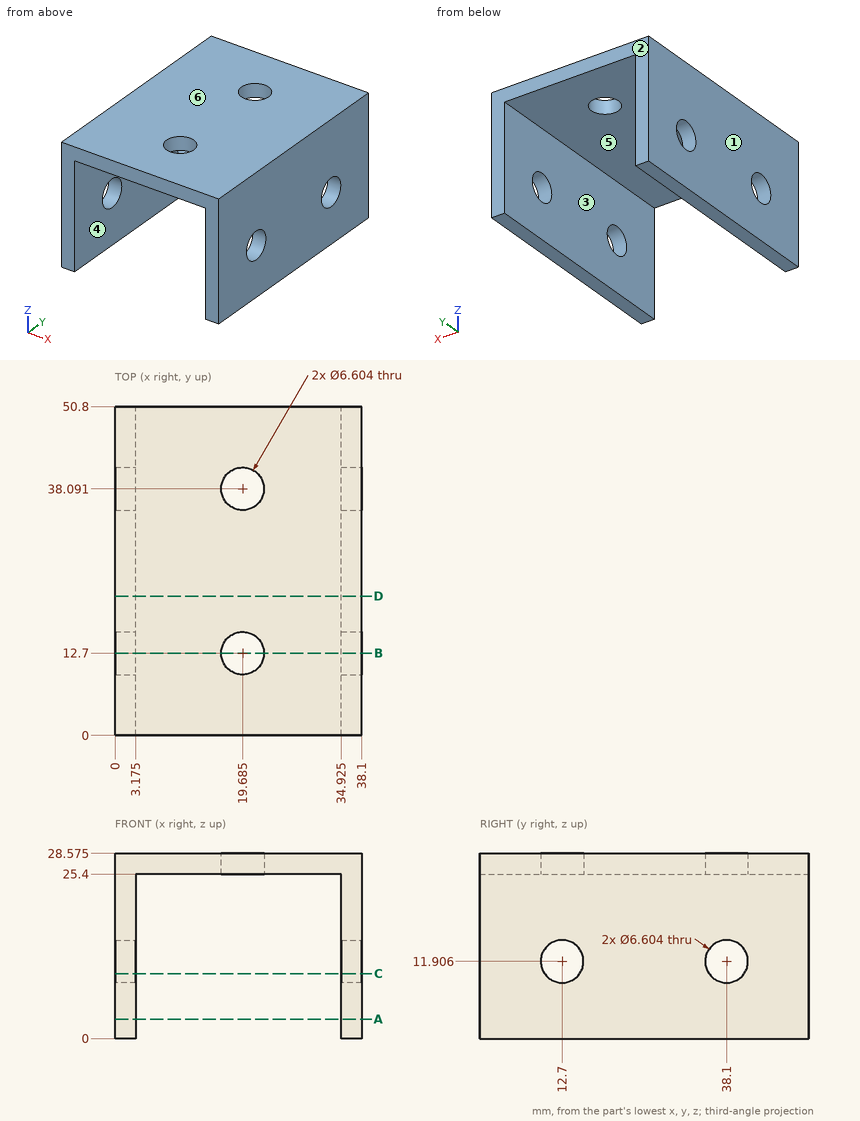
Verification items for this drawing (mm, ordinates from the low corner). A direction names the side the tool comes from. Give positions to 0.01 mm unless a question says otherwise; leave off trailing zeros. Loops run counter-clockwise (first coordinate to the right, second up) from the corner with the lowest first, then second, coordinate; pieces in that order, holes last. Notation, with made-up numbers: M -2.75,38.25 L 32.25,38.25 A12 ccw 32.25,52.25 Z; hole C 48,-38.75 d8. An arc over 180 degrees is marked long. Answer as a JSON object with one key per item and string values. Group by question number.
Q1. Cross-section at C-C on z = 10. Record the cut outline in (x, y) (1 decimal), then the cut area to 3 significant figures.
Q2. Release check for a two-part mould opening along X. For the marked faces 1, 2, 3 and 4 record: released by +X, released by -X, zero draft, split by the parting line, or undercut.
Q3. Cross-section at D-D on y = 21.5. Record the cut outline in (x, z) (1 decimal).
Q4. Go/stop test with flat-tipped pins: P1, Ø5.5, axis at y = 38.1, z = 11.91, coming from the +X side; P2, Ø5, axis at x = 17, y = 44, coming from the -Z side; P3, Ø12.5, axis at y = 13.5, z = 9, coming from the +X side. Record where each tip stops, or that it passes through.
Q5. Cross-section at A-A on z = 3. Record the cut outline in (x, y) (1 decimal).
Q6. Access from +Z, -Z, +X, -X, +Y, -Y to the whole of each face (thin tool, end or side, straight path). Record for the marked faces 5 and 6.
Q7. Cross-section at B-B on y = 12.7. Record the cut outline in (x, z) (1 decimal).
Q8. Material ranges on line 1 along X through (y, z) = (23.5, 8.5) (1 decimal); line 2 along Y through (x, z) = (36, 13.25); line 3 along Z through (x, y) = (2, 38) (1 decimal), recorded low to high. Write a range as [from, to].
Evaluation:
{
 "1": {"outline": "M 0,0 L 3.2,0 L 3.2,10 L 0,10 Z; M 0,15.4 L 3.2,15.4 L 3.2,35.4 L 0,35.4 Z; M 0,40.8 L 3.2,40.8 L 3.2,50.8 L 0,50.8 Z; M 34.9,0 L 38.1,0 L 38.1,10 L 34.9,10 Z; M 34.9,15.4 L 38.1,15.4 L 38.1,35.4 L 34.9,35.4 Z; M 34.9,40.8 L 38.1,40.8 L 38.1,50.8 L 34.9,50.8 Z", "area": "254 mm2"},
 "2": {"face 1": "released by -X", "face 2": "zero draft", "face 3": "undercut", "face 4": "undercut"},
 "3": {"outline": "M 0,0 L 3.2,0 L 3.2,25.4 L 34.9,25.4 L 34.9,0 L 38.1,0 L 38.1,28.6 L 0,28.6 Z"},
 "4": {"P1": "passes through", "P2": "stops at z = 25.4", "P3": "stops at x = 38.1"},
 "5": {"outline": "M 0,0 L 3.2,0 L 3.2,50.8 L 0,50.8 Z; M 34.9,0 L 38.1,0 L 38.1,50.8 L 34.9,50.8 Z"},
 "6": {"face 5": "-Z, +Y, -Y", "face 6": "+Z, +X, -X, +Y, -Y"},
 "7": {"outline": "M 0,0 L 3.2,0 L 3.2,8.6 L 0,8.6 Z; M 0,15.2 L 3.2,15.2 L 3.2,25.4 L 16.4,25.4 L 16.4,28.6 L 0,28.6 Z; M 23,25.4 L 34.9,25.4 L 34.9,15.2 L 38.1,15.2 L 38.1,28.6 L 23,28.6 Z; M 34.9,0 L 38.1,0 L 38.1,8.6 L 34.9,8.6 Z"},
 "8": {"line 1": "x = [0, 3.2], [34.9, 38.1]", "line 2": "y = [0, 9.68], [15.72, 35.08], [41.12, 50.8]", "line 3": "z = [0, 8.6], [15.2, 28.6]"}
}
